Build history of the part. All positions in model axes, mm. Coordinates: 2 decimals unless noted, no trailing zeros. Write each loop counter-clockwise with the first axis right and the second up, starting at its lowest first coordinate (ties: lowest second). Pieces come first, ordered by that corner, then holes.
from build123d import *

# Parameters (mm, degrees)
SKETCH1_W                       = 60.325
SKETCH1_H                       = 36.5125
EXTRUDE1_DEPTH                  = 1.5875
CHAMFER1_SIZE                   = 1.5875
F_6_CLEARANCE_HOLE1_D           = 3.7973
F_6_CLEARANCE_HOLE1_DEPTH       = 25.4
F_6_CLEARANCE_HOLE1_CSINK_D     = 7.14375
F_6_CLEARANCE_HOLE1_CSINK_ANGLE = 82
F_6_CLEARANCE_HOLE1_TIP         = 1.140824014


with BuildPart() as part:
    # Sketch1 → Extrude1 (new body, symmetric)
    with BuildSketch(Plane.XY):
        Rectangle(SKETCH1_W, SKETCH1_H)
    extrude(amount=EXTRUDE1_DEPTH, both=True)

    # Chamfer1
    chamfer1_edges = [part.edges().sort_by_distance(p)[0] for p in [
        (0, 18.25625, -1.5875),
    ]]
    chamfer(chamfer1_edges, length=CHAMFER1_SIZE)

    # #6 Clearance Hole1
    with Locations(Plane(origin=(-20.6375, -0.79375, 1.5875), x_dir=(1, 0, 0), z_dir=(0, 0, 1))):
        with Locations((0, 0), (41.275, 0)):
            CounterSinkHole(F_6_CLEARANCE_HOLE1_D / 2, F_6_CLEARANCE_HOLE1_CSINK_D / 2, depth=F_6_CLEARANCE_HOLE1_DEPTH, counter_sink_angle=F_6_CLEARANCE_HOLE1_CSINK_ANGLE)
            with Locations((0, 0, -(F_6_CLEARANCE_HOLE1_DEPTH + F_6_CLEARANCE_HOLE1_TIP / 2))):  # 118° drill point
                Cone(0, F_6_CLEARANCE_HOLE1_D / 2, F_6_CLEARANCE_HOLE1_TIP, mode=Mode.SUBTRACT)


solid = part.part
(1) Two-plate mould, pull along Y, no slides. Class faces 1 (the flat face through (0, 18.256, 1)), 2 (the cylindrical face through (-18.74, -0.71, -0.97)), 3 (the flat face through (0, -18.256, 0)): pulls with the +Y half, pulls with the -Y half, needs draft (parallel to the pull), parting line crosses it, or undercut.
(2) Slice it at A-A, the plane z = 0.75. List the corners of the cut face in (x, y), and give its area (3 significant figures).
(3) Probe L1, parallel to X at y = -0.5, z = -0.5; L2, parallel to Y at x = 21, z = 0.05; L3, parallel to Y at x = -19, z = 0.1. List the from-to ranges inside material, lowest first.
(4) Slice it at B-B, the plane y = 0. Give the number of separate pieces and of enclosed holes in the cut face, and give its area (3 significant figures).
Results:
1. face 1: pulls with the +Y half
1. face 2: undercut
1. face 3: pulls with the -Y half
2. outline: (-30.16, -18.26) - (30.16, -18.26) - (30.16, 18.26) - (-30.16, 18.26) - close; hole circle Ø5.69 at (-20.64, -0.79); hole circle Ø5.69 at (20.64, -0.79)
2. area: 2,150 mm2
3. L1: x = -30.16 to -22.51, -18.76 to 18.76, 22.51 to 30.16
3. L2: y = -18.26 to -3, 1.41 to 18.26
3. L3: y = -18.26 to -2.38, 0.79 to 18.26
4. separate pieces: 3
4. enclosed holes: 0
4. area: 163 mm2
